```python
from build123d import *

# Parameters (mm, degrees)
SKETCH1_R           = 21.5
BOSS_EXTRUDE1_DEPTH = 4
CHAMFER1_SIZE       = 0.5


with BuildPart() as part:
    # Sketch1 → Boss-Extrude1 (new body)
    with BuildSketch(Plane(origin=(0, 0, 0), x_dir=(1, 0, 0), z_dir=(0, 1, 0))):
        with Locations(Location((0, 0, 0), (0, 0, 270))):
            Circle(SKETCH1_R)
        with BuildLine():
            Line((5.384776311, 17), (-5.384776311, 17))
            ThreePointArc((-5.384776311, 17), (-6.91551004, 16.69551813), (-8.213203436, 15.828427125))
            Line((-8.213203436, 15.828427125), (-15.828427125, 8.213203436))
            ThreePointArc((-15.828427125, 8.213203436), (-16.69551813, 6.91551004), (-17, 5.384776311))
            Line((-17, 5.384776311), (-17, -5.384776311))
            ThreePointArc((-17, -5.384776311), (-16.69551813, -6.91551004), (-15.828427125, -8.213203436))
            Line((-15.828427125, -8.213203436), (-8.213203436, -15.828427125))
            ThreePointArc((-8.213203436, -15.828427125), (-6.91551004, -16.69551813), (-5.384776311, -17))
            Line((-5.384776311, -17), (5.384776311, -17))
            ThreePointArc((5.384776311, -17), (6.91551004, -16.69551813), (8.213203436, -15.828427125))
            Line((8.213203436, -15.828427125), (15.828427125, -8.213203436))
            ThreePointArc((15.828427125, -8.213203436), (16.69551813, -6.91551004), (17, -5.384776311))
            Line((17, -5.384776311), (17, 5.384776311))
            ThreePointArc((17, 5.384776311), (16.69551813, 6.91551004), (15.828427125, 8.213203436))
            Line((15.828427125, 8.213203436), (8.213203436, 15.828427125))
            ThreePointArc((8.213203436, 15.828427125), (6.91551004, 16.69551813), (5.384776311, 17))
        make_face(mode=Mode.SUBTRACT)
    extrude(amount=BOSS_EXTRUDE1_DEPTH)

    # Chamfer1
    chamfer1_edges = [part.edges().sort_by_distance(p)[0] for p in [
        (-6.91551004, 0, -16.69551813),
        (-12.02081528, 0, -12.02081528),
        (0, 0, -21.5),
        (-16.69551813, 0, -6.91551004),
        (-17, 0, 0),
        (-16.69551813, 0, 6.91551004),
        (-12.02081528, 0, 12.02081528),
        (-6.91551004, 0, 16.69551813),
        (0, 0, 17),
        (6.91551004, 0, 16.69551813),
        (12.02081528, 0, 12.02081528),
        (16.69551813, 0, 6.91551004),
        (17, 0, 0),
        (16.69551813, 0, -6.91551004),
        (12.02081528, 0, -12.02081528),
        (6.91551004, 0, -16.69551813),
        (0, 0, -17),
        (-6.91551004, 4, -16.69551813),
        (-12.02081528, 4, -12.02081528),
        (-16.69551813, 4, -6.91551004),
        (-17, 4, 0),
        (-16.69551813, 4, 6.91551004),
        (-12.02081528, 4, 12.02081528),
        (-6.91551004, 4, 16.69551813),
        (0, 4, 17),
        (6.91551004, 4, 16.69551813),
        (12.02081528, 4, 12.02081528),
        (16.69551813, 4, 6.91551004),
        (17, 4, 0),
        (16.69551813, 4, -6.91551004),
        (12.02081528, 4, -12.02081528),
        (6.91551004, 4, -16.69551813),
        (0, 4, -17),
        (0, 4, -21.5),
    ]]
    chamfer(chamfer1_edges, length=CHAMFER1_SIZE)


solid = part.part
```
Can you work these out from the model? Positions are in its coordinate system, mm. A direction names the side the tool comes from. Coordinates: 2 decimals unless noted, no trailing zeros. Loops run counter-clockwise (first coordinate to the right, second up) from the corner with the lowest first, then second, coordinate; pieces in that order, holes last.
1) I need wall thicknesses on probe 1 along X at (y, z) = (1.7, -11.5); probe 2 along Z at (x, y) = (-7, 3.1); probe 3 along Z at (x, y) = (9, 2.6). Which ranges of each line are inside material? Lowest first, please.
2) Which directions (+Z, -Z, +X, -X, +Y, -Y) give clear straight access to the entire face, cutting with the end or side of a thin tool? Please do faces 1 (the flat face through (-12.147, 0.247, -12.253)), 2 (the conical face through (-6.97, 3.7, -16.89)), 3 (the cylindrical face through (-6.9, 2, -16.7)).
3) Imagine slicing it at C-C on z = 0. List the corners of the cut face in (x, y) for me.
4) For pin 1 (2 mm diameter, centred on x = -12, y = 1.5, fed in from -Z); pin 2 (1 mm diameter, centred on y = 1, z = -15.5, fed in from +X); pin 3 (0.9 mm diameter, centred on x = -1.5, y = 1.5, fed in from +Z); pin 4 (1 mm diameter, centred on x = -15, z = 1.5, fed in from +Y), each with a flat end and sliding along its axis, tell me the tip position at first contact or that it passes through.
5) Imagine slicing it at A-A on x = 0. List the corners of the cut face in (y, z) for me, plus the area to 3 significant figures.
6) Imagine slicing it at B-B on y = 1.15. List the corners of the cut face in (x, z) for me.
Completed:
1. probe 1: x = -18.17 to -12.54, 12.54 to 18.17
1. probe 2: z = -20.33 to -16.66, 16.66 to 20.33
1. probe 3: z = -19.53 to -15.04, 15.04 to 19.53
2. face 1: -Y
2. face 2: +Y
2. face 3: +Y, -Y
3. outline: (-21.5, 0.5) - (-21, 0) - (-17.5, 0) - (-17, 0.5) - (-17, 3.5) - (-17.5, 4) - (-21, 4) - (-21.5, 3.5) - close; (17, 0.5) - (17.5, 0) - (21, 0) - (21.5, 0.5) - (21.5, 3.5) - (21, 4) - (17.5, 4) - (17, 3.5) - close
4. pin 1: stops at z = -18.47
4. pin 2: stops at x = 15.4
4. pin 3: stops at z = 21.47
4. pin 4: passes through
5. outline: (0, -21) - (0.5, -21.5) - (3.5, -21.5) - (4, -21) - (4, -17.5) - (3.5, -17) - (0.5, -17) - (0, -17.5) - close; (0, 17.5) - (0.5, 17) - (3.5, 17) - (4, 17.5) - (4, 21) - (3.5, 21.5) - (0.5, 21.5) - (0, 21) - close
5. area: 35.0 mm2
6. outline: circle Ø43 at (0, 0); hole (-17, -5.38) arc R4 ccw to (-15.83, -8.21) - (-8.21, -15.83) arc R4 ccw to (-5.38, -17) - (5.38, -17) arc R4 ccw to (8.21, -15.83) - (15.83, -8.21) arc R4 ccw to (17, -5.38) - (17, 5.38) arc R4 ccw to (15.83, 8.21) - (8.21, 15.83) arc R4 ccw to (5.38, 17) - (-5.38, 17) arc R4 ccw to (-8.21, 15.83) - (-15.83, 8.21) arc R4 ccw to (-17, 5.38) - close
